```python
from build123d import *

# Parameters (mm, degrees)
C_CHANNEL_120_X_12_1_DEPTH = 1700


with BuildPart() as part:
    # Sketch12 → C channel 120 X 12(1) (new body)
    with BuildSketch(Plane.ZY):
        with BuildLine():
            Line((65, 125), (0, 125))
            Line((0, 125), (0, 0))
            Line((0, 0), (65, 0))
            Line((65, 0), (65, 5.845330836))
            ThreePointArc((65, 5.845330836), (63.844151715, 8.856418565), (60.970378085, 10.320679365))
            Line((60.970378085, 10.320679365), (13.463772294, 15.313824837))
            ThreePointArc((13.463772294, 15.313824837), (8.354841396, 17.916955149), (6.3, 23.27))
            Line((6.3, 23.27), (6.3, 106.74))
            ThreePointArc((6.3, 106.74), (8.354841396, 112.093044851), (13.463772294, 114.696175163))
            Line((13.463772294, 114.696175163), (60.970378085, 119.689320635))
            ThreePointArc((60.970378085, 119.689320635), (63.844151715, 121.153581435), (65, 124.164669164))
            Line((65, 124.164669164), (65, 125))
        make_face()
    extrude(amount=C_CHANNEL_120_X_12_1_DEPTH)


solid = part.part
```
Geometry: final body of the model. Coordinates: model frame, mm. A direction names the side the tool comes from. Give positions to 0.01 mm unless a question says otherwise; leave off trailing zeros. Loops run counter-clockwise (first coordinate to the right, second up) from the corner with the lowest first, then second, coordinate; pieces in that order, holes last. Notation, with made-up numbers: (75.5, 78) -> (127.5, 78) arc R19 cw to (127.5, 102) -> close; hole circle Ø10 at (55, -9.75). An arc over 180 degrees is marked (long way). Return JSON: item names as keys, results as strings.
Item 1: Section C-C, the plane y = 48. Output: boundary loops of the cut face in (x, z), plus the area to 3 significant figures.
Filled in:
{"outline": "(-1700, 0) -> (0, 0) -> (0, 6.3) -> (-1700, 6.3) -> close", "area": "10,700 mm^2"}
Item 2: Mould query, pull axis Y, two halves, no side actions, for faces 1 (the flat face through (-838.1, 117.158, 36.885)), 2 (the flat face through (-838, 125, 33)), 3 (the flat face through (0, 54, 6)). Classes: released by +Y, released by -Y, zero draft, split by the parting line, or undercut.
Filled in:
{"face 1": "undercut", "face 2": "released by +Y", "face 3": "zero draft"}
Item 3: Access query for faces 4 (the flat face through (-838, 64, 6.3)), 5 (the flat face through (-838, 63, 0)). Directions: +Z, -Z, +X, -X, +Y, -Y. A direction counts if a zero-diameter tool reaches every point of the face in a straight line with its end or side. Return the directions, or none.
Filled in:
{"face 4": "+Z, +X, -X", "face 5": "-Z, +X, -X, +Y, -Y"}
Item 4: Section A-A, the plane z = 29. Output: boundary loops of the cut face in (x, y), plus the area to 3 significant figures.
Filled in:
{"outline": "(-1700, 0) -> (0, 0) -> (0, 13.68) -> (-1700, 13.68) -> close; (-1700, 116.33) -> (0, 116.33) -> (0, 125) -> (-1700, 125) -> close", "area": "38,000 mm^2"}
Item 5: Line query: line 1 (Y direction, x = -1165, z = 12); line 2 (Y direction, x = -975.5, z = 61); line 3 (Z direction, x = -750, y = 81). Output: solid intervals per line, ascending.
Filled in:
{"line 1": "0 to 15.61, 114.4 to 125", "line 2": "0 to 10.32, 119.69 to 125", "line 3": "0 to 6.3"}
Item 6: Section B-B, the plane x = -262. Output: boundary loops of the cut face in (y, z), plus the area to 3 significant figures.
Filled in:
{"outline": "(0, 0) -> (125, 0) -> (125, 65) -> (124.16, 65) arc R4.5 ccw to (119.69, 60.97) -> (114.7, 13.46) arc R8 cw to (106.74, 6.3) -> (23.27, 6.3) arc R8 cw to (15.31, 13.46) -> (10.32, 60.97) arc R4.5 ccw to (5.85, 65) -> (0, 65) -> close", "area": "2,030 mm^2"}
